```python
from build123d import *

# Parameters (mm, degrees)
F0_W           = 25
F0_H           = 30
F1_DEPTH       = 4
F2_W           = 25
F2_H           = 11
F3_DEPTH       = 13
F4_R           = 1.675
F5_DEPTH       = 25
F5_DEPTH_BACK  = 25
F7_DEPTH       = 6
F8_R           = 8
F9_DEPTH       = 6
F4_R_2         = 3
F10_DEPTH      = 2
F10_DEPTH_BACK = 25
F11_R          = 5
F13_DEPTH      = 2
F14_W          = 11
F14_H          = 17
F15_DEPTH      = 2
F16_R          = 1.45
F17_DEPTH      = 25
F18_T1_DEPTH   = 42
F18_T6_DEPTH   = 41.5273716251
F18_T11_DEPTH  = 41.5273716251
F18_T16_DEPTH  = 41.5273716251
F18_T21_DEPTH  = 41.5273716251


# Not quite as in the source:
# - a fillet or chamfer that OpenCascade refuses, or shapes differently, is made with other operations: its cross-section is extruded or revolved along the edge and cut away or added


with BuildPart() as f1:
    # F0 (on Top) → F1 (new body)
    with BuildSketch(Plane.XY):
        with Locations((12.5, 15)):
            Rectangle(F0_W, F0_H)
    extrude(amount=F1_DEPTH)

    # F2 (on face) → F3 (join)
    with BuildSketch(Plane.XY.offset(4)):
        with Locations((12.5, 24.5)):
            Rectangle(F2_W, F2_H)
    extrude(amount=F3_DEPTH)

    # F4 (on face) → F5 (cut, two sides)
    with BuildSketch(Plane.XY.offset(4)) as f5_sk:
        with BuildLine():
            ThreePointArc((3.325, 18.5605346784), (5, 16.8855346784), (6.675, 18.5605346784))
            ThreePointArc((6.675, 18.5605346784), (6.6602655711, 18.7822174099), (6.6163215123, 19))
            Line((6.6163215123, 19), (3.3836784877, 19))
            ThreePointArc((3.3836784877, 19), (3.3397344289, 18.7822174099), (3.325, 18.5605346784))
        make_face()
        with BuildLine():
            ThreePointArc((21.6163215123, 19), (20, 20.2355346784), (18.3836784877, 19))
            Line((18.3836784877, 19), (21.6163215123, 19))
        make_face()
        with BuildLine():
            Line((21.6163215123, 19), (18.3836784877, 19))
            ThreePointArc((18.3836784877, 19), (19.7783172685, 16.9002691073), (21.675, 18.5605346784))
            ThreePointArc((21.675, 18.5605346784), (21.6602655711, 18.7822174099), (21.6163215123, 19))
        make_face()
        with Locations((20, 3.5605346784)):
            Circle(F4_R)
        with Locations((5, 3.5605346784)):
            Circle(F4_R)
        with BuildLine():
            Line((3.3836784877, 19), (6.6163215123, 19))
            ThreePointArc((6.6163215123, 19), (5, 20.2355346784), (3.3836784877, 19))
        make_face()
    extrude(amount=-F5_DEPTH, mode=Mode.SUBTRACT)
    extrude(f5_sk.sketch, amount=F5_DEPTH_BACK, mode=Mode.SUBTRACT)

    # F6 (on face) → F7 (cut)
    with BuildSketch(Plane(origin=(0, 30, 0), x_dir=(-1, 0, 0), z_dir=(0, 1, 0))):
        with BuildLine():
            ThreePointArc((-18.5, 17), (-12.5, 11), (-6.5, 17))
            Line((-6.5, 17), (-18.5, 17))
        make_face()
    extrude(amount=-F7_DEPTH, mode=Mode.SUBTRACT)

    # F8 (on face) → F9 (cut)
    with BuildSketch(Plane.XZ.offset(-19)):
        with Locations((12.5394891948, 17)):
            Circle(F8_R)
    extrude(amount=-F9_DEPTH, mode=Mode.SUBTRACT)

    # F4 (on face) → F10 (cut, two sides)
    with BuildSketch(Plane.XY.offset(4)) as f10_sk:
        with BuildLine():
            ThreePointArc((3.3836784877, 19), (5, 20.2355346784), (6.6163215123, 19))
            Line((6.6163215123, 19), (7.9676371461, 19))
            ThreePointArc((7.9676371461, 19), (5, 21.5605346784), (2.0323628539, 19))
            Line((2.0323628539, 19), (3.3836784877, 19))
        make_face()
        with BuildLine():
            Line((2, 18.5605346784), (3.325, 18.5605346784))
            ThreePointArc((3.325, 18.5605346784), (3.3397344289, 18.7822174099), (3.3836784877, 19))
            Line((3.3836784877, 19), (2.0323628539, 19))
            ThreePointArc((2.0323628539, 19), (2.0081016529, 18.7808623453), (2, 18.5605346784))
        make_face()
        with BuildLine():
            ThreePointArc((6.6163215123, 19), (6.6602655711, 18.7822174099), (6.675, 18.5605346784))
            ThreePointArc((6.675, 18.5605346784), (5, 16.8855346784), (3.325, 18.5605346784))
            Line((3.325, 18.5605346784), (2, 18.5605346784))
            ThreePointArc((2, 18.5605346784), (5, 15.5605346784), (8, 18.5605346784))
            ThreePointArc((8, 18.5605346784), (7.9918983471, 18.7808623453), (7.9676371461, 19))
            Line((7.9676371461, 19), (6.6163215123, 19))
        make_face()
        with BuildLine():
            ThreePointArc((22.9676371461, 19), (20, 21.5605346784), (17.0323628539, 19))
            Line((17.0323628539, 19), (18.3836784877, 19))
            ThreePointArc((18.3836784877, 19), (20, 20.2355346784), (21.6163215123, 19))
            Line((21.6163215123, 19), (22.9676371461, 19))
        make_face()
        with BuildLine():
            Line((18.3836784877, 19), (17.0323628539, 19))
            ThreePointArc((17.0323628539, 19), (19.7796723331, 15.5686363313), (23, 18.5605346784))
            ThreePointArc((23, 18.5605346784), (22.9918983471, 18.7808623453), (22.9676371461, 19))
            Line((22.9676371461, 19), (21.6163215123, 19))
            ThreePointArc((21.6163215123, 19), (21.6602655711, 18.7822174099), (21.675, 18.5605346784))
            ThreePointArc((21.675, 18.5605346784), (19.7783172685, 16.9002691073), (18.3836784877, 19))
        make_face()
        with Locations((20, 3.5605346784)):
            Circle(F4_R_2)
        with Locations((20, 3.5605346784)):
            Circle(F4_R, mode=Mode.SUBTRACT)
        with Locations((5, 3.5605346784)):
            Circle(F4_R_2)
        with Locations((5, 3.5605346784)):
            Circle(F4_R, mode=Mode.SUBTRACT)
    extrude(amount=-F10_DEPTH, mode=Mode.SUBTRACT)
    extrude(f10_sk.sketch, amount=F10_DEPTH_BACK, mode=Mode.SUBTRACT)

    # F11
    f11_edges = [f1.edges().sort_by_distance(p)[0] for p in [
        (0, 0, 2),
        (25, 0, 2),
    ]]
    fillet(f11_edges, radius=F11_R)

    # F12 (on face) → F13 (join)
    with BuildSketch(Plane(origin=(0, 0, 0), x_dir=(0, -1, 0), z_dir=(-1, 0, 0))):
        Polygon((-30, 17), (-30, 0), (-19, 0), (-19, 4), (-19, 17), align=None)
    extrude(amount=F13_DEPTH)

    # F14 (on face) → F15 (join)
    with BuildSketch(Plane.YZ.offset(25)):
        with Locations((24.5, 8.5)):
            Rectangle(F14_W, F14_H)
    extrude(amount=F15_DEPTH)

    # F16 (on face) → F17 (cut)
    with BuildSketch(Plane.XY.offset(17)):
        with Locations((0.45, 25.55)):
            Circle(F16_R)
        with Locations((24.55, 25.55)):
            Circle(F16_R)
    extrude(amount=-F17_DEPTH, mode=Mode.SUBTRACT)

    # F18: fillet of radius 5 on 4 edges, made by hand

    # F18_s2 → F18_t1 (cut)
    with BuildSketch(Plane.XY.offset(-12.5)):
        with BuildLine():
            ThreePointArc((-2, 25), (-0.5355339059, 28.5355339059), (3, 30))
            Line((3, 30), (-2, 30))
            Line((-2, 30), (-2, 25))
        make_face()
        with BuildLine():
            ThreePointArc((22, 30), (25.5355339059, 28.5355339059), (27, 25))
            Line((27, 25), (27, 30))
            Line((27, 30), (22, 30))
        make_face()
    extrude(amount=F18_T1_DEPTH, mode=Mode.SUBTRACT)


with BuildPart() as f18_tool4:
    # F18_s5 → F18_t6 (new body)
    with BuildSketch(Plane.XY.offset(29.2636858126)):
        with BuildLine():
            ThreePointArc((2.0323628539, 19), (-0.8625241572, 20.7304298947), (-2, 23.905474325))
            Line((-2, 23.905474325), (-2, 19))
            Line((-2, 19), (2.0323628539, 19))
        make_face()
    extrude(amount=-F18_T6_DEPTH)

    split(bisect_by=Plane.XY.offset(4), keep=Keep.TOP)


with BuildPart() as f1_1:
    add(f1.part)

    # F18_t3: cut F18_tool4
    add(f18_tool4.part, mode=Mode.SUBTRACT)


with BuildPart() as f18_tool9:
    # F18_s10 → F18_t11 (new body)
    with BuildSketch(Plane.XY.offset(29.2636858126)):
        with BuildLine():
            ThreePointArc((2.0323628539, 19), (-0.8625241572, 20.7304298947), (-2, 23.905474325))
            Line((-2, 23.905474325), (-2, 19))
            Line((-2, 19), (2.0323628539, 19))
        make_face()
    extrude(amount=-F18_T11_DEPTH)

    split(bisect_by=Plane.YZ, keep=Keep.BOTTOM)


with BuildPart() as f1_2:
    add(f1_1.part)

    # F18_t8: cut F18_tool9
    add(f18_tool9.part, mode=Mode.SUBTRACT)


with BuildPart() as f18_tool14:
    # F18_s15 → F18_t16 (new body)
    with BuildSketch(Plane.XY.offset(29.2636858126)):
        with BuildLine():
            ThreePointArc((22.9676371461, 19), (25.8625241572, 20.7304298947), (27, 23.905474325))
            Line((27, 23.905474325), (27, 19))
            Line((27, 19), (22.9676371461, 19))
        make_face()
    extrude(amount=-F18_T16_DEPTH)

    split(bisect_by=Plane.XY.offset(4), keep=Keep.TOP)


with BuildPart() as f1_3:
    add(f1_2.part)

    # F18_t13: cut F18_tool14
    add(f18_tool14.part, mode=Mode.SUBTRACT)


with BuildPart() as f18_tool19:
    # F18_s20 → F18_t21 (new body)
    with BuildSketch(Plane.XY.offset(29.2636858126)):
        with BuildLine():
            ThreePointArc((22.9676371461, 19), (25.8625241572, 20.7304298947), (27, 23.905474325))
            Line((27, 23.905474325), (27, 19))
            Line((27, 19), (22.9676371461, 19))
        make_face()
    extrude(amount=-F18_T21_DEPTH)

    split(bisect_by=Plane.YZ.offset(25), keep=Keep.TOP)


with BuildPart() as f1_4:
    add(f1_3.part)

    # F18_t18: cut F18_tool19
    add(f18_tool19.part, mode=Mode.SUBTRACT)


solid = f1_4.part
```
Work out the finished part from the listing and answer in its coordinate system (mm). A direction names the side the tool comes from. Give positions to 0.01 mm unless a question says otherwise; leave off trailing zeros. Write each loop counter-clockwise with the first axis right and the second up, starting at its lowest first coordinate (ties: lowest second). Pieces come first, ordered by that corner, then holes.
(1) The part is cut by section B-B on z = 14.25. Write down the section's boundary in (x, y), plus the area to 3 significant figures.
Final values:
outline: (-2, 23.91) arc R5 ccw to (2.03, 19) arc R3 cw to (5.03, 21.56) - (5.03, 25) - (7.17, 25) - (7.17, 30) - (3, 30) arc R5 ccw to (-2, 25) - close; (17.83, 25) - (20.05, 25) - (20.05, 21.56) arc R3 cw to (22.97, 19) arc R5 ccw to (27, 23.91) - (27, 25) arc R5 ccw to (22, 30) - (17.83, 30) - close; hole circle Ø2.9 at (0.45, 25.55); hole circle Ø2.9 at (24.55, 25.55)
area: 130 mm2
(2) Flat-ended cylindrical pins translate along their axes: pin 1 Ø2 at (x, y) = (20, 18.56) entering from -Z (1 decimal); pin 2 Ø10 at (y, z) = (19, 12) entering from -X; pin 3 Ø1.2 at (y, z) = (10, 1.5) entering from -X; pin 4 Ø4.5 at (y, z) = (10, 2) entering from +X. Find the tip coordinate at first contact, or state that the pin passes through.
Final values:
pin 1: passes through
pin 2: stops at x = -2
pin 3: stops at x = 0
pin 4: stops at x = 25
(3) Straight lines are drawn through the part: line 1 (Y direction, x = 20, z = 0.75); line 2 (Y direction, x = 14.25, z = 6.5); line 3 (Z direction, x = 11.5, y = 18.5). For each, find the intervals that lie inside material, in ascending order.
Final values:
line 1: y = 0 to 1.89, 5.24 to 16.89, 20.24 to 30
line 2: y = 19 to 30
line 3: z = 0 to 4
(4) The part is cut by section D-D on y = 2.5. Write down the section's boundary in (x, z), plus the area to 3 significant figures.
Final values:
outline: (0.67, 0) - (3.7, 0) - (3.7, 2) - (2.19, 2) - (2.19, 4) - (0.67, 4) - close; (6.3, 0) - (18.7, 0) - (18.7, 2) - (17.19, 2) - (17.19, 4) - (7.81, 4) - (7.81, 2) - (6.3, 2) - close; (21.3, 0) - (24.33, 0) - (24.33, 4) - (22.81, 4) - (22.81, 2) - (21.3, 2) - close
area: 61.8 mm2
(5) The part is cut by section C-C on x = 24. Write down the section's boundary in (y, z).
Final values:
outline: (2, 0) - (24.21, 0) - (24.21, 17) - (19.32, 17) - (19.32, 4) - (2, 4) - close; (26.89, 0) - (29.58, 0) - (29.58, 17) - (26.89, 17) - close
(6) Which of the six approach directions +Z, -Z, +X, -X, +Y, -Y give full straight-line access (tool end or side, diameter ignored) to faces 5 (the cylindrical face through (17.619, 1.735, 3.014)), 6 (the flat face through (12, 19, 6)), 7 (the flat face through (0, 12, 2)), 8 (the flat face through (12.5, 25, 10.6))?
Final values:
face 5: +Z
face 6: +Z, +X, -X, -Y
face 7: +Z, -Z, -X, -Y
face 8: +Z, -Y
(7) The part is cut by section A-A on z = 8.25. Write down the section's boundary in (x, y).
Final values:
outline: (-2, 23.91) arc R5 ccw to (2.03, 19) arc R3 cw to (7.97, 19) - (17.03, 19) arc R3 cw to (22.97, 19) arc R5 ccw to (27, 23.91) - (27, 25) arc R5 ccw to (22, 30) - (3, 30) arc R5 ccw to (-2, 25) - close; hole circle Ø2.9 at (0.45, 25.55); hole circle Ø2.9 at (24.55, 25.55)
(8) The mould has two halves that part along Y. Classify faces 1 (the flat face through (12, 0, 2)), 2 (the flat face through (12, 15, 0)), 3 (the cylindrical face through (21.547, 2.919, 1.014)), 4 (the flat face through (6, 17, 2)): pulls with the +Y half, pulls with the -Y half, needs draft (parallel to the pull), parting line crosses it, or undercut.
Final values:
face 1: pulls with the -Y half
face 2: needs draft
face 3: undercut
face 4: undercut
